from build123d import *

# Parameters (mm, degrees)
SKETCH1_W                                       = 10
SKETCH1_H                                       = 10
BOSS_EXTRUDE1_DEPTH                             = 75
M3X0_5_TAPPED_HOLE1_D                           = 2.5
M3X0_5_TAPPED_HOLE1_DEPTH                       = 7.5
M3X0_5_TAPPED_HOLE1_TIP                         = 0.751075774
M3X0_5_TAPPED_HOLE2_D                           = 2.5
M3X0_5_TAPPED_HOLE2_DEPTH                       = 7.5
M3X0_5_TAPPED_HOLE2_TIP                         = 0.751075774
CSK_FOR_M3_OVAL_HEAD_MACHINE_SCREW1_D           = 3.4
CSK_FOR_M3_OVAL_HEAD_MACHINE_SCREW1_CSINK_D     = 6.3
CSK_FOR_M3_OVAL_HEAD_MACHINE_SCREW1_CSINK_ANGLE = 90
M3X0_5_TAPPED_HOLE3_D                           = 2.5


with BuildPart() as part:
    # Sketch1 → Boss-Extrude1 (new body)
    with BuildSketch(Plane.XY):
        with Locations((32.5, -32.5)):
            Rectangle(SKETCH1_W, SKETCH1_H)
    extrude(amount=BOSS_EXTRUDE1_DEPTH)

    # M3x0.5 Tapped Hole1
    with Locations(Plane.XY.offset(75)):
        with Locations((32.5, -32.5)):
            Hole(M3X0_5_TAPPED_HOLE1_D / 2, depth=M3X0_5_TAPPED_HOLE1_DEPTH)
            with Locations((0, 0, -(M3X0_5_TAPPED_HOLE1_DEPTH + M3X0_5_TAPPED_HOLE1_TIP / 2))):  # 118° drill point
                Cone(0, M3X0_5_TAPPED_HOLE1_D / 2, M3X0_5_TAPPED_HOLE1_TIP, mode=Mode.SUBTRACT)

    # M3x0.5 Tapped Hole2
    with Locations(Plane(origin=(0, 0, 0), x_dir=(-1, 0, 0), z_dir=(0, 0, -1))):
        with Locations((-32.5, -32.5)):
            Hole(M3X0_5_TAPPED_HOLE2_D / 2, depth=M3X0_5_TAPPED_HOLE2_DEPTH)
            with Locations((0, 0, -(M3X0_5_TAPPED_HOLE2_DEPTH + M3X0_5_TAPPED_HOLE2_TIP / 2))):  # 118° drill point
                Cone(0, M3X0_5_TAPPED_HOLE2_D / 2, M3X0_5_TAPPED_HOLE2_TIP, mode=Mode.SUBTRACT)

    # CSK for M3 Oval Head Machine Screw1 (through all)
    with Locations(Plane(origin=(27.5, -32.5, 37.5), x_dir=(0, 0, -1), z_dir=(-1, 0, 0))):
        with Locations((0, 0)):
            CounterSinkHole(CSK_FOR_M3_OVAL_HEAD_MACHINE_SCREW1_D / 2, CSK_FOR_M3_OVAL_HEAD_MACHINE_SCREW1_CSINK_D / 2, counter_sink_angle=CSK_FOR_M3_OVAL_HEAD_MACHINE_SCREW1_CSINK_ANGLE)

    # M3x0.5 Tapped Hole3 (through all)
    with Locations(Plane(origin=(0, -27.5, 0), x_dir=(-1, 0, 0), z_dir=(0, 1, 0))):
        with Locations((-32.5, 65), (-32.5, 10)):
            Hole(M3X0_5_TAPPED_HOLE3_D / 2)


solid = part.part
Build history of the part. All positions in model axes, mm. A direction names the side the tool comes from. Give positions to 0.01 mm unless a question says otherwise; leave off trailing zeros. Loops run counter-clockwise (first coordinate to the right, second up) from the corner with the lowest first, then second, coordinate; pieces in that order, holes last. Notation, with made-up numbers: (-38.75, 42.25) - (-22.75, 42.25) arc R26 ccw to (-22.75, 63.25) - close; hole circle Ø10 at (-36, -25.5). An arc over 180 degrees is marked (long way). Write item = value, one per line. Start each with the question number.
1) Tool access for faces 4 (the conical face through (32.38, -32.32, 8.12)), 5 (the cylindrical face through (31.345, -32.979, 71.198)): list every direction of +Z, -Z, +X, -X, +Y, -Y with a clear straight run to the whole face (end or side of a thin tool).
2) Pull direction X, two halves, no side cores. Call faces 1 (the flat face through (27.5, -29, 37)), 2 (the flat face through (32, -37.5, 37)), 3 (the cylindrical face through (33.69, -32.12, 3.8)): +X half, -X half, draft (parallel to the pull), parting line (faces both ways), or undercut.
3) Probe probe 1 along Z at (x, y) = (32.5, -32.5); probe 2 along Z at (x, y) = (35.25, -32.5); probe 3 along Y at (x, z) = (35.25, 37.5). List the from-to ranges inside material, lowest first. Write a range as from..to.
4) Drop flat-ended pins along their axis: pin 1 Ø2 at (x, y) = (32.5, -32.5) entering from +Z; pin 2 Ø5 at (x, y) = (32, -31.5) entering from -Z; pin 3 Ø5.5 at (y, z) = (-32.5, 37.5) entering from -X. Give the stop position or say it passes through.
5) Band-saw the part on A-A on z = 65. Give the cut face in (x, y).
Final values:
q1.face_4 = -Z
q1.face_5 = +Z
q2.face_1 = -X half
q2.face_2 = draft
q2.face_3 = undercut
q3.probe_1 = 8.25..8.75, 11.25..35.8, 39.2..63.75, 66.25..66.75
q3.probe_2 = 0..35.8, 39.2..75
q3.probe_3 = -37.5..-34.2, -30.8..-27.5
q4.pin_1 = 67.35
q4.pin_2 = 0
q4.pin_3 = 27.9
q5.outline = (27.5, -37.5) - (31.25, -37.5) - (31.25, -27.5) - (27.5, -27.5) - close; (33.75, -37.5) - (37.5, -37.5) - (37.5, -27.5) - (33.75, -27.5) - close
